```python
from build123d import *

# Parameters (mm, degrees)
SKETCH1_R           = 2
SKETCH1_R_2         = 2.5
BOSS_EXTRUDE1_DEPTH = 3
FILLET1_R           = 1


with BuildPart() as part:
    # Sketch1 → Boss-Extrude1 (new body)
    with BuildSketch(Plane(origin=(0, 0, 0), x_dir=(1, 0, 0), z_dir=(0, 1, 0))):
        with BuildLine():
            Line((-5.5, 2), (-5.5, -2))
            ThreePointArc((-5.5, -2), (-4.328427125, -4.828427125), (-1.5, -6))
            Line((-1.5, -6), (39.5, -6))
            ThreePointArc((39.5, -6), (42.328427125, -4.828427125), (43.5, -2))
            Line((43.5, -2), (43.5, 2))
            ThreePointArc((43.5, 2), (42.328427125, 4.828427125), (39.5, 6))
            Line((39.5, 6), (-1.5, 6))
            ThreePointArc((-1.5, 6), (-4.328427125, 4.828427125), (-5.5, 2))
        make_face()
        with Locations(Location((0, 0, 0), (0, 0, 270))):
            Circle(SKETCH1_R, mode=Mode.SUBTRACT)
        with Locations(Location((38, 0, 0), (0, 0, 270))):
            Circle(SKETCH1_R, mode=Mode.SUBTRACT)
        with Locations(Location((19.050336346, -0.050336346, 0), (0, 0, 270))):
            Circle(SKETCH1_R_2, mode=Mode.SUBTRACT)
    extrude(amount=BOSS_EXTRUDE1_DEPTH)

    # Fillet1
    fillet1_edges = [part.edges().sort_by_distance(p)[0] for p in [
        (-4.328427125, 3, -4.828427125),
        (-5.5, 3, 0),
        (-4.328427125, 3, 4.828427125),
        (19, 3, 6),
        (42.328427125, 3, 4.828427125),
        (43.5, 3, 0),
        (42.328427125, 3, -4.828427125),
        (19, 3, -6),
    ]]
    fillet(fillet1_edges, radius=FILLET1_R)


solid = part.part
```
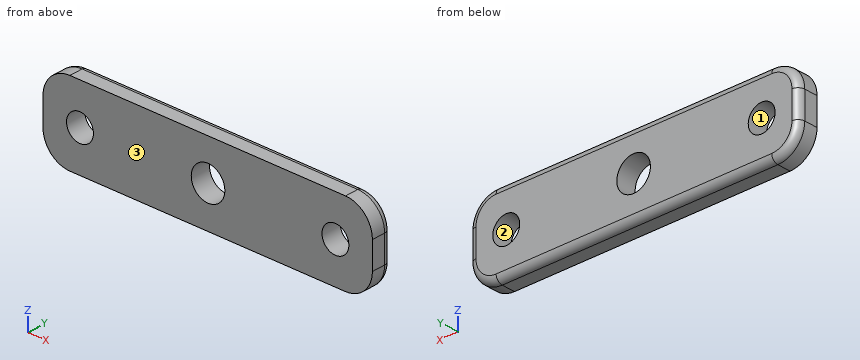
Geometry check sheet. Reference: the model listing, model coordinates, mm. Face numbers are marked on the shaded views. Round coordinates to 2 decimals unless told otherwise and drop trailing zeros. Loops run counter-clockwise (first coordinate to the right, second up) from the corner with the lowest first, then second, coordinate; pieces in that order, holes last. Notation, with made-up numbers: M 7,85.5 L 43,85.5 A21 cw 43,122.5 Z; hole C 35,-36.75 d7. An arc over 180 degrees is marked long. Return JSON: item names as keys, results as strings. Group by question number.
(1) Scan lines: line 1 along X through (y, z) = (1.75, 0); line 2 along X through (y, z) = (2.65, -1); line 3 along Z through (x, y) = (20.5, 1.1). Record each from-to range of solid material in increasing order. Write a range as [from, to].
(2) Section check A-A, the plane x = 0. Enter the section's corners in (y, z).
(3) Mould release check, pull along Z, two halves, no side actions. Record for the marked faces 1, 2 and 3: pulls with the +Z half, pulls with the -Z half, needs draft (parallel to the pull), parting line crosses it, or undercut.
(4) Section check B-B, the plane y = 0.8. Enter the section's corners in (x, z), and give its area (3 significant figures).
(5) Section check D-D, the plane x = 17. Enter the section's corners in (y, z), and give its area (3 significant figures).
(6) Section check C-C, the plane z = 0. Enter the section's corners in (x, y), and give its area (3 significant figures).
Data:
{
 "1": {"line 1": "[-5.5, -2], [2, 16.55], [21.55, 36], [40, 43.5]", "line 2": "[-5.26, -1.73], [1.73, 16.78], [21.32, 36.27], [39.73, 43.26]", "line 3": "[-6, -1.99], [2.09, 6]"},
 "2": {"outline": "M 0,-6 L 2,-6 A1 ccw 3,-5 L 3,-2 L 0,-2 Z; M 0,2 L 3,2 L 3,5 A1 ccw 2,6 L 0,6 Z"},
 "3": {"face 1": "undercut", "face 2": "undercut", "face 3": "needs draft"},
 "4": {"outline": "M -5.5,-2 A4 ccw -1.5,-6 L 39.5,-6 A4 ccw 43.5,-2 L 43.5,2 A4 ccw 39.5,6 L -1.5,6 A4 ccw -5.5,2 Z; hole C 0,0 d4; hole C 19.05,0.05 d5; hole C 38,0 d4", "area": "529 mm²"},
 "5": {"outline": "M 0,-6 L 2,-6 A1 ccw 3,-5 L 3,-1.38 L 0,-1.38 Z; M 0,1.48 L 3,1.48 L 3,5 A1 ccw 2,6 L 0,6 Z", "area": "27.0 mm²"},
 "6": {"outline": "M -5.5,0 L -2,0 L -2,3 L -4.5,3 A1 ccw -5.5,2 Z; M 2,0 L 16.55,0 L 16.55,3 L 2,3 Z; M 21.55,0 L 36,0 L 36,3 L 21.55,3 Z; M 40,0 L 43.5,0 L 43.5,2 A1 ccw 42.5,3 L 40,3 Z", "area": "108 mm²"}
}
